The listing builds one solid part. Answer for the finished solid, in the listing's coordinates (mm). Face numbers are marked on the shaded views. A direction names the side the tool comes from. Round coordinates to 2 decimals unless told otherwise and drop trailing zeros. Write each loop counter-clockwise with the first axis right and the second up, starting at its lowest first coordinate (ties: lowest second). Pieces come first, ordered by that corner, then holes.
Item 1: Find the intervals of material crossed by probe 1 along Y at (x, z) = (0, 25); probe 2 along X at (y, z) = (41, 37.5); probe 3 along X at (y, z) = (41.5, 45), in increasing order.
Item 2: Each of these flat-tipped pins is pushed along its axis until it touches: pin 1 (5.5 mm diameter, centred on x = -14.59, y = -5, fed in from -Z); pin 2 (12 mm diameter, centred on x = -2, z = 46, fed in from +Y); pin 3 (3 mm diameter, centred on y = 14.5, z = 10, fed in from +X); pin 4 (4.5 mm diameter, centred on x = -38, y = 29.88, fed in from -Z). Where does it stop, or does it pass through?
Item 3: Find section A-A on y = 0. Give the vertices of the cut face in (x, z), then the cut area to 3 significant figures.
Item 4: Find section B-B on z = 47.5. Give the vertices of the cut face in (x, y), then the cut area to 3 significant figures.
Item 5: For a pull along Y with two mould halves and no side action, classify the marked faces 5, 6, 7 and 8 as +Y half, -Y half, draft (parallel to the pull), parting line (faces both ways), or undercut.
Item 6: Find section C-C on z = 68.5. Give the number of separate pieces and of enclosed holes in the cut face, then the cut area to 3 significant figures.
Item 7: A tool of negligible diameter and unlimited length cuts with its end or side. For the marked faces 1, 2, 3 and 4, from which of +Z, -Z, +X, -X, +Y, -Y can it reach the whole face along a straight path? Write none if from no direction.
```python
from build123d import *

# Parameters (mm, degrees)
BOSS_EXTRUDE1_DEPTH = 35
BOSS_EXTRUDE2_START = -20
SKETCH2_R           = 55
SKETCH2_R_2         = 39.161040577
BOSS_EXTRUDE2_DEPTH = 40
SKETCH4_R           = 55
BOSS_EXTRUDE3_DEPTH = 20
SKETCH5_R           = 3
CUT_EXTRUDE1_DEPTH  = 20
SKETCH6_R           = 2.5
CUT_EXTRUDE3_DEPTH  = 109.050914096
SKETCH8_R           = 2.25
SKETCH8_R_2         = 2.2
SKETCH8_W           = 40.596274726
SKETCH8_H           = 19.795896112
CUT_EXTRUDE5_DEPTH  = 30


with BuildPart() as part:
    # Sketch1 → Boss-Extrude1 (new body)
    with BuildSketch(Plane.XY):
        with BuildLine():
            add(Edge.make_bspline(
                [(-38, 20), (-28.167603026, 32.926551341), (0, 39.5)],
                knots=[0, 0, 0, 1, 1, 1], degree=2))
            add(Edge.make_bspline(
                [(0, 39.5), (28.167603026, 32.926551341), (38, 20)],
                knots=[0, 0, 0, 1, 1, 1], degree=2))
            Line((38, 20), (38, 10))
            Line((38, 10), (54.083269132, 10))
            ThreePointArc((54.083269132, 10), (0, 55), (-54.083269132, 10))
            Line((-54.083269132, 10), (-38, 10))
            Line((-38, 10), (-38, 20))
        make_face()
    extrude(amount=BOSS_EXTRUDE1_DEPTH)

    # Sketch2 → Boss-Extrude2 (add)
    with BuildSketch(Plane.XY.offset(35).offset(BOSS_EXTRUDE2_START)):
        with Locations(Location((0, 0, 0), (0, 0, 169.524318304))):
            Circle(SKETCH2_R)
        Circle(SKETCH2_R_2, mode=Mode.SUBTRACT)
    extrude(amount=BOSS_EXTRUDE2_DEPTH)

    # Sketch4 → Boss-Extrude3 (add)
    with BuildSketch(Plane.XY.offset(55)):
        with Locations(Location((0, 0, 0), (0, 0, 169.524318304))):
            Circle(SKETCH4_R)
    extrude(amount=BOSS_EXTRUDE3_DEPTH)

    # Sketch5 → Cut-Extrude1 (cut)
    with BuildSketch(Plane.XY.offset(75)):
        Circle(SKETCH5_R)
    extrude(amount=-CUT_EXTRUDE1_DEPTH, mode=Mode.SUBTRACT)

    # Sketch6 → Cut-Extrude3 (cut, through all)
    with BuildSketch(Plane.XY.offset(75)):
        with Locations((-38, 29.880895352)):
            Circle(SKETCH6_R)
        with Locations((-22, 41.266508356)):
            Circle(SKETCH6_R)
        with Locations((0, 47.25)):
            Circle(SKETCH6_R)
        with Locations((22, 41.266508356)):
            Circle(SKETCH6_R)
        with Locations((38, 29.880895352)):
            Circle(SKETCH6_R)
    extrude(amount=-CUT_EXTRUDE3_DEPTH, mode=Mode.SUBTRACT)

    # Sketch8 → Cut-Extrude5 (cut)
    with BuildSketch(Plane.XY.offset(75)):
        with Locations((-14.589613301, 5)):
            Circle(SKETCH8_R)
        with Locations((-14.589613301, -5)):
            Circle(SKETCH8_R_2)
        with Locations((35.189613301, 5)):
            Circle(SKETCH8_R_2)
        with Locations((35.189613301, -5)):
            Circle(SKETCH8_R_2)
        with Locations((10.298137363, 0.002051944)):
            Rectangle(SKETCH8_W, SKETCH8_H)
    extrude(amount=-CUT_EXTRUDE5_DEPTH, mode=Mode.SUBTRACT)


solid = part.part
```
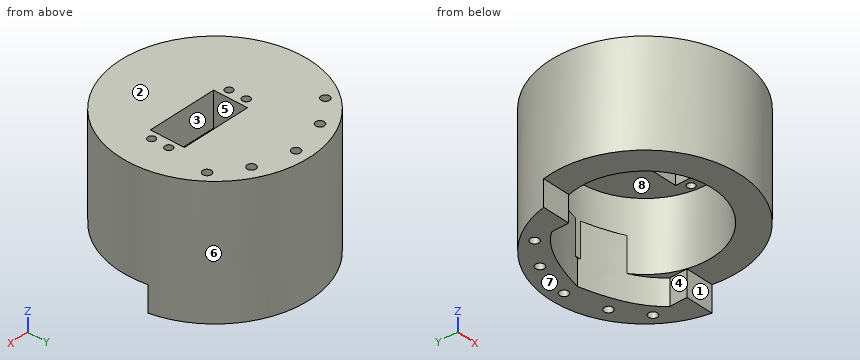
Check values:
1. probe 1: y = -55 to -39.16, 39.16 to 44.75, 49.75 to 55
1. probe 2: x = -36.66 to -24.49, -19.51 to 19.51, 24.49 to 36.66
1. probe 3: x = -36.09 to -24.49, -19.51 to 19.51, 24.49 to 36.09
2. pin 1: stops at z = 55
2. pin 2: stops at y = 55
2. pin 3: stops at x = 53.44
2. pin 4: passes through
3. outline: (-55, 15) - (-39.16, 15) - (-39.16, 55) - (-10, 55) - (-10, 75) - (-55, 75) - close; (30.6, 55) - (39.16, 55) - (39.16, 15) - (55, 15) - (55, 75) - (30.6, 75) - close
3. area: 2,660 mm2
4. outline: circle Ø110 at (0, 0); hole circle Ø5 at (-38, 29.88); hole circle Ø78.32 at (0, 0); hole circle Ø5 at (-22, 41.27); hole circle Ø5 at (0, 47.25); hole circle Ø5 at (22, 41.27); hole circle Ø5 at (38, 29.88)
4. area: 4,590 mm2
5. face 5: undercut
5. face 6: parting line
5. face 7: draft
5. face 8: undercut
6. separate pieces: 1
6. enclosed holes: 10
6. area: 8,540 mm2
7. face 1: -Z, +X, -X, -Y
7. face 2: +Z, +X, -X, +Y, -Y
7. face 3: +Z, -Z
7. face 4: -Z, -Y
